Model file for the job. Use its own axes, mm. Give positions to 0.01 mm unless a question says otherwise; leave off trailing zeros. Order: outer loops, then holes, each group sorted by start corner. A loop starts at its lowest first (then second) coordinate and runs counter-clockwise, first axis right, second up. Notation, with made-up numbers: (45.25, 59.25) -> (74.25, 59.25) arc R24 cw to (74.25, 77.25) -> close; hole circle Ø1 at (33.25, -28). An arc over 180 degrees is marked (long way). Answer in a Markdown table with one row per item. Add a question column.
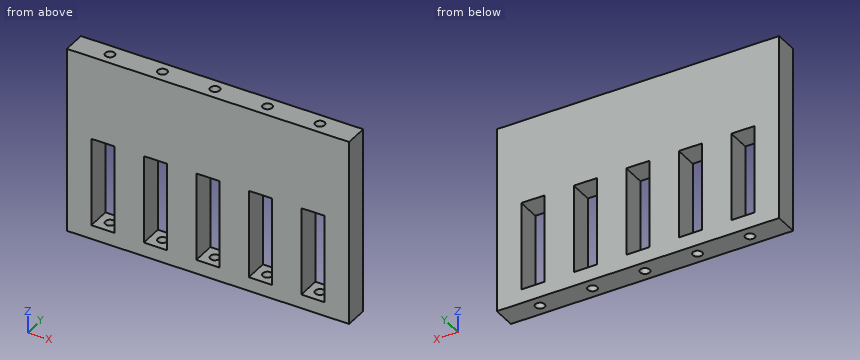
from build123d import *

# Parameters (mm, degrees)
SKETCH1_W           = 121
SKETCH1_H           = 80
BOSS_EXTRUDE1_DEPTH = 10
SKETCH2_W           = 10
SKETCH2_H           = 68
CUT_EXTRUDE1_DEPTH  = 10
SKETCH7_R           = 2
CUT_EXTRUDE4_DEPTH  = 108.099253032
SKETCH8_W           = 100
SKETCH8_H           = 30
BOSS_EXTRUDE4_DEPTH = 10


with BuildPart() as part:
    # Sketch1 → Boss-Extrude1 (new body)
    with BuildSketch(Plane(origin=(0, 0, 0), x_dir=(1, 0, 0), z_dir=(0, 1, 0))):
        with Locations((10, 40)):
            Rectangle(SKETCH1_W, SKETCH1_H)
    extrude(amount=BOSS_EXTRUDE1_DEPTH)

    # Sketch2 → Cut-Extrude1 (cut)
    with BuildSketch(Plane(origin=(0, 10, 0), x_dir=(1, 0, 0), z_dir=(0, 1, 0))):
        with Locations((-35, 40)):
            Rectangle(SKETCH2_W, SKETCH2_H)
        with Locations((-12.5, 40)):
            Rectangle(SKETCH2_W, SKETCH2_H)
        with Locations((10, 40)):
            Rectangle(SKETCH2_W, SKETCH2_H)
        with Locations((32.5, 40)):
            Rectangle(SKETCH2_W, SKETCH2_H)
        with Locations((55, 40)):
            Rectangle(SKETCH2_W, SKETCH2_H)
    extrude(amount=-CUT_EXTRUDE1_DEPTH, mode=Mode.SUBTRACT)

    # Sketch7 → Cut-Extrude4 (cut, through all)
    with BuildSketch(Plane.XY):
        with Locations((-35, 5)):
            Circle(SKETCH7_R)
        with Locations((-12.5, 5)):
            Circle(SKETCH7_R)
        with Locations((10, 5)):
            Circle(SKETCH7_R)
        with Locations((32.5, 5)):
            Circle(SKETCH7_R)
        with Locations((55, 5)):
            Circle(SKETCH7_R)
    extrude(amount=-CUT_EXTRUDE4_DEPTH, mode=Mode.SUBTRACT)

    # Sketch8 → Boss-Extrude4 (add)
    with BuildSketch(Plane(origin=(0, 10, 0), x_dir=(1, 0, 0), z_dir=(0, 1, 0))):
        with Locations((10, 21)):
            Rectangle(SKETCH8_W, SKETCH8_H)
    extrude(amount=-BOSS_EXTRUDE4_DEPTH)


solid = part.part
Item 1: Saw through at B-B on z = -71. List the corners of the cut face in (x, y), plus the area to 3 significant figures.
Item 2: Pin check, flat tip, straight feed: pin 1 Ø3 at (x, y) = (55, 5) entering from +Z. Stop position of the tip, or through.
Item 3: Wall check: line 1 (X direction, y = 0.5, z = -50); line 2 (Z direction, x = 36, y = 2.5); line 3 (Y direction, x = -35, z = -78.1). Give the ranges that are in metal, low to high.
Item 4: Saw through at A-A on x = -12.5. List the corners of the cut face in (y, z).
Evaluation:
| question | item | result |
|---|---|---|
| 1 | outline | (-50.5, 0) -> (-40, 0) -> (-40, 10) -> (-50.5, 10) -> close; (-30, 0) -> (-17.5, 0) -> (-17.5, 10) -> (-30, 10) -> close; (-7.5, 0) -> (5, 0) -> (5, 10) -> (-7.5, 10) -> close; (15, 0) -> (27.5, 0) -> (27.5, 10) -> (15, 10) -> close; (37.5, 0) -> (50, 0) -> (50, 10) -> (37.5, 10) -> close; (60, 0) -> (70.5, 0) -> (70.5, 10) -> (60, 10) -> close |
| 1 | area | 710 mm2 |
| 2 | pin 1 | stops at z = -6 |
| 3 | line 1 | x = -50.5 to -40, -30 to -17.5, -7.5 to 5, 15 to 27.5, 37.5 to 50, 60 to 70.5 |
| 3 | line 2 | z = -80 to -74, -36 to 0 |
| 3 | line 3 | y = 0 to 3, 7 to 10 |
| 4 | outline | (0, -80) -> (3, -80) -> (3, -74) -> (0, -74) -> close; (0, -36) -> (10, -36) -> (10, 0) -> (7, 0) -> (7, -6) -> (3, -6) -> (3, 0) -> (0, 0) -> close; (7, -80) -> (10, -80) -> (10, -74) -> (7, -74) -> close |
